The model under review builds one solid part; all positions refer to its coordinate system, in mm. A direction names the side the tool comes from. Give positions to 0.01 mm unless a question says otherwise; leave off trailing zeros. Loops run counter-clockwise (first coordinate to the right, second up) from the corner with the lowest first, then second, coordinate; pieces in that order, holes last. Notation, with made-up numbers: (-3, 38) - (56, 38) arc R27 cw to (56, 57) - close; hole circle Ø10 at (4.5, 10). An arc over 180 degrees is marked (long way). Return JSON: item names as keys, results as strings. Group by question number.
from build123d import *

# Parameters (mm, degrees)
SKETCH2_W           = 145
SKETCH2_H           = 200
BOSS_EXTRUDE1_DEPTH = 7
SKETCH5_R           = 2.25
SKETCH5_R_2         = 2.2
CUT_EXTRUDE1_DEPTH  = 33
SKETCH6_R           = 4
BOSS_EXTRUDE3_DEPTH = 50
SKETCH7_R           = 2.25
CUT_EXTRUDE2_DEPTH  = 58


with BuildPart() as part:
    # Sketch2 → Boss-Extrude1 (new body)
    with BuildSketch(Plane(origin=(0, 0, 0), x_dir=(1, 0, 0), z_dir=(0, 1, 0))):
        Rectangle(SKETCH2_W, SKETCH2_H)
    extrude(amount=BOSS_EXTRUDE1_DEPTH)

    # Sketch5 → Cut-Extrude1 (cut, through all)
    with BuildSketch(Plane(origin=(0, 32, 0), x_dir=(1, 0, 0), z_dir=(0, 1, 0))):
        with Locations((-68, 45)):
            Circle(SKETCH5_R)
        with Locations((-68, -40)):
            Circle(SKETCH5_R)
        with Locations((-68, -90)):
            Circle(SKETCH5_R_2)
        with Locations((68, -90)):
            Circle(SKETCH5_R_2)
        with Locations((68, -40)):
            Circle(SKETCH5_R)
        with Locations((68, 45)):
            Circle(SKETCH5_R)
    extrude(amount=-CUT_EXTRUDE1_DEPTH, mode=Mode.SUBTRACT)

    # Sketch6 → Boss-Extrude3 (add)
    with BuildSketch(Plane.XZ):
        with BuildLine():
            ThreePointArc((-58, 44), (-62, 40), (-58, 36))
            Line((-58, 36), (-58, 44))
        make_face()
        with BuildLine():
            Line((-58, 44), (-58, 36))
            ThreePointArc((-58, 36), (-55.171572875, 37.171572875), (-54, 40))
            ThreePointArc((-54, 40), (-55.171572875, 42.828427125), (-58, 44))
        make_face()
        with BuildLine():
            ThreePointArc((-54, 90), (-60.828427125, 92.828427125), (-58, 86))
            Line((-58, 86), (-58, 90))
            Line((-58, 90), (-54, 90))
        make_face()
        with BuildLine():
            Line((-58, 90), (-58, 86))
            ThreePointArc((-58, 86), (-55.171572875, 87.171572875), (-54, 90))
            Line((-54, 90), (-58, 90))
        make_face()
        with Locations((58, 90)):
            Circle(SKETCH6_R)
        with Locations((-58, -20)):
            Circle(SKETCH6_R)
        with Locations((58, -20)):
            Circle(SKETCH6_R)
        with Locations((58, 40)):
            Circle(SKETCH6_R)
    extrude(amount=BOSS_EXTRUDE3_DEPTH)

    # Sketch7 → Cut-Extrude2 (cut, through all)
    with BuildSketch(Plane.XZ.offset(50)):
        with Locations((-58, 90)):
            Circle(SKETCH7_R)
        with Locations((-58, 40)):
            Circle(SKETCH7_R)
        with Locations((-58, -20)):
            Circle(SKETCH7_R)
        with Locations((58, -20)):
            Circle(SKETCH7_R)
        with Locations((58, 40)):
            Circle(SKETCH7_R)
        with Locations((58, 90)):
            Circle(SKETCH7_R)
    extrude(amount=-CUT_EXTRUDE2_DEPTH, mode=Mode.SUBTRACT)


solid = part.part
Item 1: For L1, parallel to Z at x = -58, y = -34; L2, parallel to X at y = 2, z = -45; L3, parallel to Y at x = 62, z = 46, list the stretches that pass through material, from the lowest coordinate up. Write a range as from..to.
Item 2: For P1, Ø4, axis at x = -68, z = 90, coming from the +Y side; P2, Ø10, axis at x = 50.5, z = 2, coming from the -Y side; P3, Ø7, axis at x = -58, z = 90, coming from the +Y side; P4, Ø1, axis at y = -10.5, z = -19.5, coming from the -X side, all flat-tipped, find the tip position at first contact; note any pin that passes through.
Item 3: Take a section at D-D (z = -20). State the section outline as (x, y) points, then the cut area to 3 significant figures.
Item 4: Take a section at B-B (x = 68). State the section outline as (y, z) points.
Item 5: Tool access review of faces 1 (the face through (59.846, -24.65, 86.451)), 2 (the face through (-65.9, 3.55, 89.34)): name each direction out of +Z, -Z, +X, -X, +Y, -Y from which nothing blocks a thin tool from reaching the whole face with its end or side.
Item 6: Take a section at A-A (y = -22.5). State how many separate pieces and enclosed holes the cut face has, then the cut area to 3 significant figures.
Item 7: Mouldability with a two-part tool opening along Z and no side actions: class faces 3 (the face through (-1, 7, -1)), 4 (the face through (-1, 3, 100)), 5 (the face through (67.71, 3.55, -47.23)) as +Z half, -Z half, draft (parallel to the pull), parting line (faces both ways), or undercut.
Item 8: Take a section at C-C (z = -45). State the section outline as (x, y) points, then the cut area to 3 significant figures.
Check sheet entries:
{
 "1": {"L1": "z = -24..-22.25, -17.75..-16, 36..37.75, 42.25..44, 86..87.75, 92.25..94", "L2": "x = -72.5..-70.25, -65.75..65.75, 70.25..72.5", "L3": "y = 0..7"},
 "2": {"P1": "passes through", "P2": "stops at y = 0", "P3": "stops at y = 7", "P4": "stops at x = -62"},
 "3": {"outline": "(-72.5, 0) - (-62, 0) - (-62, -50) - (-60.25, -50) - (-60.25, 7) - (-72.5, 7) - close; (-55.75, -50) - (-54, -50) - (-54, 0) - (54, 0) - (54, -50) - (55.75, -50) - (55.75, 7) - (-55.75, 7) - close; (60.25, -50) - (62, -50) - (62, 0) - (72.5, 0) - (72.5, 7) - (60.25, 7) - close", "area": "1,300 mm^2"},
 "4": {"outline": "(0, -100) - (7, -100) - (7, -47.25) - (0, -47.25) - close; (0, -42.75) - (7, -42.75) - (7, 37.75) - (0, 37.75) - close; (0, 42.25) - (7, 42.25) - (7, 87.8) - (0, 87.8) - close; (0, 92.2) - (7, 92.2) - (7, 100) - (0, 100) - close"},
 "5": {"face 1": "-Y", "face 2": "+Y, -Y"},
 "6": {"separate pieces": "6", "enclosed holes": "6", "area": "206 mm^2"},
 "7": {"face 3": "draft", "face 4": "+Z half", "face 5": "undercut"},
 "8": {"outline": "(-72.5, 0) - (-70.25, 0) - (-70.25, 7) - (-72.5, 7) - close; (-65.75, 0) - (65.75, 0) - (65.75, 7) - (-65.75, 7) - close; (70.25, 0) - (72.5, 0) - (72.5, 7) - (70.25, 7) - close", "area": "952 mm^2"}
}
